```python
from build123d import *

# Parameters (mm, degrees)
F0_W     = 101.6
F0_H     = 44.45
F1_DEPTH = 63.5
F3_DEPTH = 127.001
F5_DEPTH = 127.001
F6_R     = 2.54
F8_DEPTH = 6.35
F9_R     = 5.08


# Not quite as in the source:
# - a pattern or mirror of a feature is missing from the dataset's text; its kind, count and spacing are read off the source's solid


with BuildPart() as f1:
    # F0 (on Front) → F1 (new body, symmetric)
    with BuildSketch(Plane.XZ):
        Rectangle(F0_W, F0_H)
    extrude(amount=F1_DEPTH, both=True)

    # F2 (on face) → F3 (cut, through all)
    with BuildSketch(Plane.XZ.offset(63.5)):
        Polygon((-50.8, -15.875), (-12.7, -15.875), (-12.7, -3.175), (-38.1, 22.225), (-50.8, 22.225), align=None)
    f3 = extrude(amount=-F3_DEPTH, mode=Mode.SUBTRACT)

    # F3_copies: F3 across plane
    add(f3.mirror(Plane(origin=(0, 0, 0), x_dir=(0, 0, 1), z_dir=(1, 0, 0))), mode=Mode.SUBTRACT)

    # F4 (on face) → F5 (cut, through all)
    with BuildSketch(Plane.XZ.offset(63.5)):
        Polygon((30.861, 22.225), (-30.861, 22.225), (-5.461, -3.175), (-5.461, -10.8996083293), (0, -13.4461144505), (5.461, -10.8996083293), (5.461, -3.175), align=None)
    extrude(amount=-F5_DEPTH, mode=Mode.SUBTRACT)

    # F6
    f6_edges = [f1.edges().sort_by_distance(p)[0] for p in [
        (-38.1, 0, 22.225),
        (-30.861, 0, 22.225),
        (30.861, 0, 22.225),
        (38.1, 0, 22.225),
    ]]
    fillet(f6_edges, radius=F6_R)

    # F7 (on face) → F8 (cut, through all)
    with BuildSketch(Plane(origin=(0, 0, -22.225), x_dir=(1, 0, 0), z_dir=(0, 0, -1))):
        with BuildLine():
            Line((-25.4, 45.72), (-50.8, 45.72))
            Line((-50.8, 45.72), (-50.8, 38.1))
            Line((-50.8, 38.1), (-25.4, 38.1))
            ThreePointArc((-25.4, 38.1), (-21.59, 41.91), (-25.4, 45.72))
        make_face()
        with BuildLine():
            Line((-25.4, -38.1), (-50.8, -38.1))
            Line((-50.8, -38.1), (-50.8, -45.72))
            Line((-50.8, -45.72), (-25.4, -45.72))
            ThreePointArc((-25.4, -45.72), (-21.59, -41.91), (-25.4, -38.1))
        make_face()
    f8 = extrude(amount=-F8_DEPTH, mode=Mode.SUBTRACT)

    # F8_copies: F8 across plane
    add(f8.mirror(Plane(origin=(0, 0, 0), x_dir=(0, 0, 1), z_dir=(1, 0, 0))), mode=Mode.SUBTRACT)

    # F9
    f9_edges = [f1.edges().sort_by_distance(p)[0] for p in [
        (-50.8, -63.5, -19.05),
        (-50.8, 63.5, -19.05),
        (50.8, -63.5, -19.05),
        (50.8, 63.5, -19.05),
        (-50.8, -45.72, -19.05),
        (-50.8, 38.1, -19.05),
        (-50.8, 45.72, -19.05),
        (-50.8, -38.1, -19.05),
        (50.8, 45.72, -19.05),
        (50.8, -45.72, -19.05),
        (50.8, -38.1, -19.05),
        (50.8, 38.1, -19.05),
    ]]
    fillet(f9_edges, radius=F9_R)


solid = f1.part
```
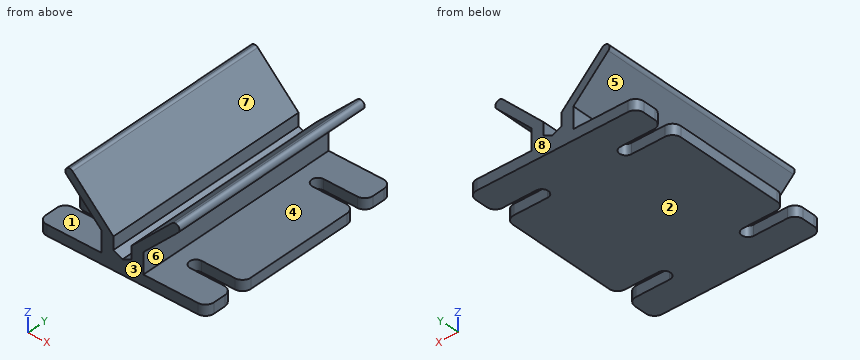
Input: part model. Units: mm. Frame: model coordinates. Face numbers are marked on the shaded views. A direction names the side the tool comes from. Coordinates: 2 decimals unless noted, no trailing zeros. Loops run counter-clockwise (first coordinate to the right, second up) from the corner with the lowest first, then second, coordinate; pieces in that order, holes last.
Q1. Section B-B, the plane x = 23. Return the cut outline in (y, z) (3 decimals), and give its area (3 significant figures).
Results are:
outline: (-63.5, -22.225) - (-44.869, -22.225) - (-44.869, -15.875) - (-63.5, -15.875) - close; (-63.5, 7.125) - (63.5, 7.125) - (63.5, 14.364) - (-63.5, 14.364) - close; (-38.951, -22.225) - (38.951, -22.225) - (38.951, -15.875) - (-38.951, -15.875) - close; (44.869, -22.225) - (63.5, -22.225) - (63.5, -15.875) - (44.869, -15.875) - close
area: 1,650 mm2
Q2. Set-up query: the marked faces 5, 6, 7 and 8. Return all of +Z, -Z, +X, -X, +Y, -Y with unobstructed straight access to the full face (end or side cutting, diameter ignored); none if empty.
Results are:
face 5: -X, +Y, -Y
face 6: +X, +Y, -Y
face 7: +Z, +Y, -Y
face 8: +Z, -Z, +X, -X, +Y
Q3. Section A-A, the plane x = -40.5. Return the cut outline in (y, z) (3 decimals).
Results are:
outline: (-63.5, -22.225) - (-45.72, -22.225) - (-45.72, -15.875) - (-63.5, -15.875) - close; (-38.1, -22.225) - (38.1, -22.225) - (38.1, -15.875) - (-38.1, -15.875) - close; (45.72, -22.225) - (63.5, -22.225) - (63.5, -15.875) - (45.72, -15.875) - close
Q4. Mould query, pull axis Z, two halves, no side actions, for the marked faces 1, 2, 3 and 4. Classes: +Z half, -Z half, draft (parallel to the pull), parting line (faces both ways), or undercut.
Results are:
face 1: undercut
face 2: -Z half
face 3: draft
face 4: undercut
Q5. Contact query for flat-ended pins moving along their axis: pin 1 (1 mm diameter, centred on x = -21.5, y = 5, fed in from +Z); pin 2 (4 mm diameter, centred on y = -17.5, z = -10, fed in from +X); pin 3 (2 mm diameter, centred on y = 7.5, z = 3, fed in from -X) (3 decimals). Output: stop coordinate, or through.
Results are:
pin 1: stops at z = 13.36
pin 2: stops at x = 12.7
pin 3: stops at x = -19.875
Q6. Section D-D, the plane z = 7.5. Return the cut outline in (x, y) (3 decimals), and give its area (3 significant figures).
Results are:
outline: (-23.375, -63.5) - (-16.136, -63.5) - (-16.136, 63.5) - (-23.375, 63.5) - close; (16.136, -63.5) - (23.375, -63.5) - (23.375, 63.5) - (16.136, 63.5) - close
area: 1,840 mm2
Q7. Section C-C, the plane y = 20.5. Return the cut outline in (x, z) (3 decimals).
Results are:
outline: (-50.8, -22.225) - (50.8, -22.225) - (50.8, -15.875) - (12.7, -15.875) - (12.7, -3.175) - (33.764, 17.889) arc R2.54 ccw to (31.968, 22.225) - (31.913, 22.225) arc R2.54 ccw to (30.117, 21.481) - (5.461, -3.175) - (5.461, -10.9) - (0, -13.446) - (-5.461, -10.9) - (-5.461, -3.175) - (-30.117, 21.481) arc R2.54 ccw to (-31.913, 22.225) - (-31.968, 22.225) arc R2.54 ccw to (-33.764, 17.889) - (-12.7, -3.175) - (-12.7, -15.875) - (-50.8, -15.875) - close
Q8. Line query: line 1 along Y through (x, z) = (31.5, -19.5); line 2 along X through (y, z) = (-48, -8); line 3 along Z through (x, y) = (17, 5) (3 decimals). Output: solid intervals per line, ascending.
Results are:
line 1: y = -63.5 to -45.72, -38.1 to 38.1, 45.72 to 63.5
line 2: x = -12.7 to -5.46, 5.46 to 12.7
line 3: z = -22.225 to -15.875, 1.125 to 8.364
